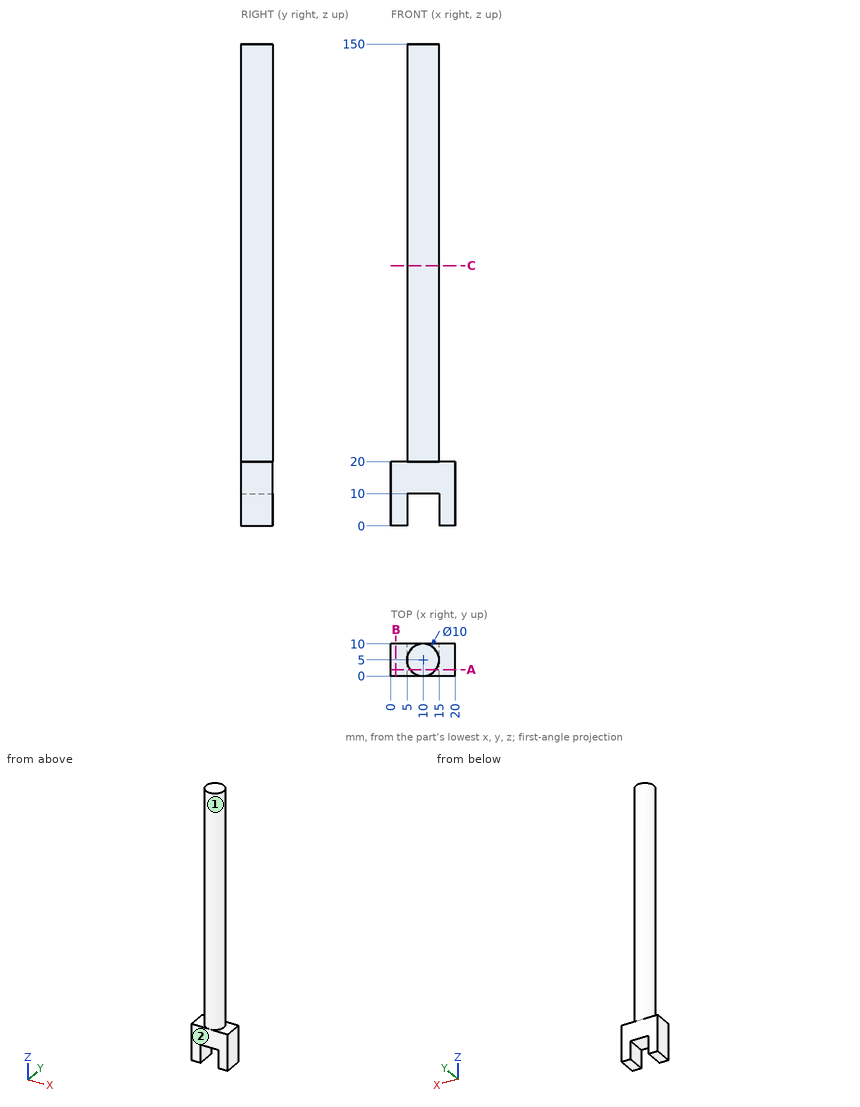
The figure shows three views and two pictorial views of one solid part (mm, origin at its lowest corner). Answer the questions. A direction names the side the tool comes from. Round coordinates to 2 decimals unless told otherwise and drop trailing zeros. Write each loop counter-clockwise with the first axis right and the second up, starting at its lowest first coordinate (ties: lowest second). Pieces come first, ordered by that corner, then holes. Notation, with made-up numbers: (-28.5, -23) - (-2.5, -23) arc R24 cw to (-2.5, 4) - close; hole circle Ø5 at (66.25, 84.5). An arc over 180 degrees is marked (long way). Answer in a Markdown table with one row per item. Add a question column.
1. A cutting plane is placed at B-B, the plane x = 1.5. Determine the outline of the cut face in (y, z).
2. A cutting plane is placed at C-C, the plane z = 81. Determine the outline of the cut face in (x, y).
3. Find the intervals of material crossed by line 1 along Z through (x, y) = (12.5, 4.5); line 2 along Z through (x, y) = (1.25, 1.75); line 3 along X through (y, z) = (4.5, 61), in increasing order. Write a range as from..to.
4. For the marked faces 1 and 2, determine the directions among +Z, -Z, +X, -X, +Y, -Y from which every point of the face is accessible in a straight line to the end or side of a thin tool.
5. A cutting plane is placed at A-A, the plane y = 2. Determine the outline of the cut face in (x, z).
6. Given pin 1 (5 mm diameter, centred on x = 3, z = 128, fed in from +Y); pin 2 (4 mm diameter, centred on x = 4, z = 45, fed in from -Y); pin 3 (6 mm diameter, centred on y = 9, z = 133, fed in from +X); pin 4 (4 mm diameter, centred on x = 3, y = 9, fed in from -Z), each flat-ended and moving along its own axis, determine where each tip first touches the part or whether it passes through.
Worked out:
| question | item | result |
|---|---|---|
| 1 | outline | (0, 0) - (10, 0) - (10, 20) - (0, 20) - close |
| 2 | outline | circle Ø10 at (10, 5) |
| 3 | line 1 | 10..150 |
| 3 | line 2 | 0..20 |
| 3 | line 3 | 5.03..14.97 |
| 4 | face 1 | +Z |
| 4 | face 2 | +Z, -Z, +X, -X, -Y |
| 5 | outline | (0, 0) - (5, 0) - (5, 10) - (15, 10) - (15, 0) - (20, 0) - (20, 20) - (14, 20) - (14, 150) - (6, 150) - (6, 20) - (0, 20) - close |
| 6 | pin 1 | y = 7.18 |
| 6 | pin 2 | y = 2 |
| 6 | pin 3 | x = 14.9 |
| 6 | pin 4 | z = 0 |
